Input: part model. Units: mm. Frame: model coordinates. Coordinates: 2 decimals unless noted, no trailing zeros. Write each loop counter-clockwise with the first axis right and the second up, starting at its lowest first coordinate (ties: lowest second). Pieces come first, ordered by that corner, then holes. Notation, with made-up numbers: (33, -10.5) - (64, -10.5) arc R26 ccw to (64, 8.5) - close; hole circle Ø7 at (4, 74). An arc over 180 degrees is marked (long way). Put each result on its own line as item: value. Start each with the question number.
1. Cut plane A-A, the plane x = 67.5. Return loops of the section in (y, z).
2. Pin query (flat end, axial travel): pin 1 (1.9 mm diameter, centred on x = 57.5, z = 0, fed in from -Y); pin 2 (3 mm diameter, centred on x = 1, y = 30.5, fed in from -Z); pin 3 (1.5 mm diameter, centred on x = 52.5, z = 3, fed in from +Y); pin 4 (1.2 mm diameter, centred on y = 17, z = 2.5, fed in from +X). Return the tip coordinate at first contact, or that it passes through.
3. Cut plane C-C, the plane x = 9.5. Return loops of the section in (y, z).
4. Line query: line 1 (X direction, y = 1.15, z = 0); line 2 (Z direction, x = 67.5, y = 1.6); line 3 (X direction, y = 16, z = 2.25). Output: solid intervals per line, ascending.
5. Cut plane B-B, the plane y = 12. Return loops of the section in (x, z), and give its area (4 significant figures).
from build123d import *

# Parameters (mm, degrees)
SKETCH_1_R      = 1.6
EXTRUDE_1_DEPTH = 5
SKETCH_2_W      = 105
SKETCH_2_H      = 2.5
EXTRUDE_2_DEPTH = 30
FILLET_4_R      = 2
FILLET_5_R      = 2


with BuildPart() as part:
    # 草图1 → 凸台-拉伸1 (new body)
    with BuildSketch(Plane(origin=(0, 0, 0), x_dir=(1, 0, 0), z_dir=(0, 1, 0))):
        Polygon((72.5, -4), (-72.5, -4), (-72.5, 2.9), (-52.5, 2.9), (-52.5, -1.5), (52.5, -1.5), (52.5, 2.9), (72.5, 2.9), align=None)
        with Locations(Location((-67.5, 0, 0), (0, 0, 270))):
            Circle(SKETCH_1_R, mode=Mode.SUBTRACT)
        with Locations(Location((-57.5, 0, 0), (0, 0, 270))):
            Circle(SKETCH_1_R, mode=Mode.SUBTRACT)
        with Locations(Location((67.5, 0, 0), (0, 0, 90))):
            Circle(SKETCH_1_R, mode=Mode.SUBTRACT)
        with Locations(Location((57.5, 0, 0), (0, 0, 90))):
            Circle(SKETCH_1_R, mode=Mode.SUBTRACT)
    extrude(amount=EXTRUDE_1_DEPTH)

    # 草图2 → 凸台-拉伸2 (add)
    with BuildSketch(Plane(origin=(0, 5, 0), x_dir=(1, 0, 0), z_dir=(0, 1, 0))):
        with Locations((0, -2.75)):
            Rectangle(SKETCH_2_W, SKETCH_2_H)
    extrude(amount=EXTRUDE_2_DEPTH)

    # 圆角4
    fillet_4_edges = [part.edges().sort_by_distance(p)[0] for p in [
        (72.5, 2.5, 4),
        (-72.5, 2.5, 4),
        (72.5, 2.5, -2.9),
        (-72.5, 2.5, -2.9),
        (52.5, 2.5, -2.9),
        (-52.5, 2.5, -2.9),
        (-52.5, 2.5, 1.5),
        (52.5, 2.5, 1.5),
        (52.5, 35, 2.75),
        (-52.5, 35, 2.75),
    ]]
    fillet(fillet_4_edges, radius=FILLET_4_R)

    # 圆角5
    fillet_5_edges = [part.edges().sort_by_distance(p)[0] for p in [
        (-52.5, 5, 2.75),
        (52.5, 5, 2.75),
    ]]
    fillet(fillet_5_edges, radius=FILLET_5_R)


solid = part.part
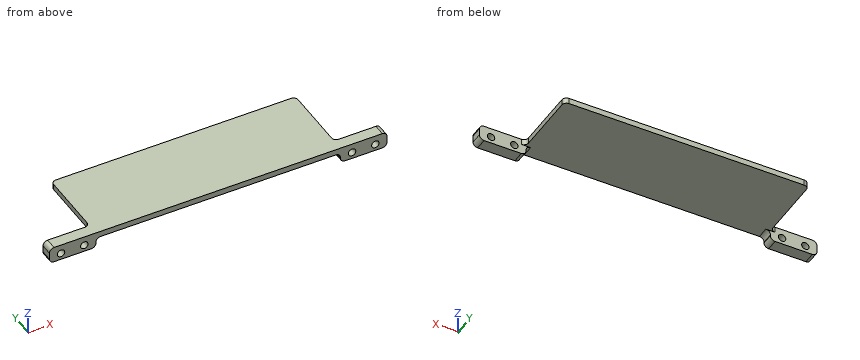
Report:
1. outline: (0, -2.9) - (5, -2.9) - (5, -1.6) - (0, -1.6) - close; (0, 1.6) - (5, 1.6) - (5, 4) - (0, 4) - close
2. pin 1: passes through
2. pin 2: stops at z = 1.5
2. pin 3: stops at y = 34.56
2. pin 4: stops at x = 52.5
3. outline: (0, 1.5) - (35, 1.5) - (35, 4) - (0, 4) - close
4. line 1: x = -72.5 to -69.1, -65.9 to -59.1, -55.9 to -52.44, 52.44 to 55.9, 59.1 to 65.9, 69.1 to 72.5
4. line 2: z = -2.9 to -1.6, 1.6 to 4
4. line 3: x = -52.5 to 52.5
5. outline: (-52.5, 1.5) - (52.5, 1.5) - (52.5, 4) - (-52.5, 4) - close
5. area: 262.5 mm^2
